```python
from build123d import *

# Parameters (mm, degrees)
SKETCH2_R           = 3.5
BOSS_EXTRUDE1_DEPTH = 3


with BuildPart() as part:
    # Sketch2 → Boss-Extrude1 (new body)
    with BuildSketch(Plane.XY):
        Polygon((-9.966299499, 13.71), (-6.966299499, 13.71), (-6.966299499, 10.71), (-3.966299499, 10.71), (-3.966299499, 13.71), (-0.966299499, 13.71), (-0.966299499, 10.71), (2.033700501, 10.71), (2.033700501, 13.71), (5.033700501, 13.71), (5.033700501, 10.71), (8.033700501, 10.71), (8.033700501, 13.71), (11.033700501, 13.71), (11.033700501, -22.29), (8.033700501, -22.29), (8.033700501, -19.29), (7.033700501, -19.29), (7.033700501, -6.29), (-5.966299499, -6.29), (-5.966299499, -19.29), (-6.966299499, -19.29), (-6.966299499, -22.29), (-9.966299499, -22.29), align=None)
        with Locations((0.533700501, 3.71)):
            Circle(SKETCH2_R, mode=Mode.SUBTRACT)
    extrude(amount=BOSS_EXTRUDE1_DEPTH)


solid = part.part
```
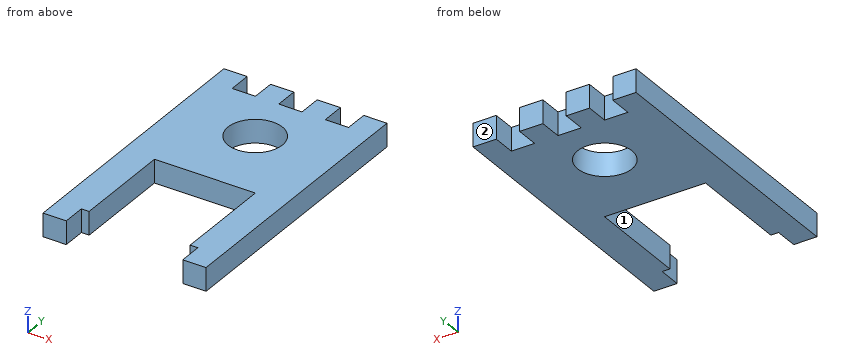
Geometry check sheet. Reference: the model listing, model coordinates, mm. Face numbers are marked on the shaded views. A direction names the side the tool comes from. Coordinates: 2 decimals unless noted, no trailing zeros. Order: outer loops, then holes, each group sorted by start corner. A loop starts at its lowest first (then second) coordinate and runs counter-clockwise, first axis right, second up. Notation, with made-up numbers: (51, 45.25) - (78, 45.25) arc R14 cw to (78, 72.25) - close; hole circle Ø8 at (28, -29). An arc over 180 degrees is marked (long way). Answer in a Markdown table with one row per item. Add a question column.
1. Material ranges on L1, parallel to X at y = 12, z = 0.5; L2, parallel to X at y = -9, z = 2.7; L3, parallel to X at y = 3.5, z = 1.4, recorded low to high. Write a range as [from, to].
2. Section check B-B (z = 1.95). Enter the section's corners in (x, y), plus the area to 3 significant figures.
3. Section check C-C (y = -10.5). Enter the section's corners in (x, z).
4. Access from +Z, -Z, +X, -X, +Y, -Y to the whole of each face (thin tool, end or side, straight path). Record for the marked faces 1 and 2.
5. Gauge pin test, flat ends, axial feed: pin 1 Ø8 at (x, y) = (0.53, 3.71) entering from +Z; pin 2 Ø1 at (x, z) = (-4.5, 0.5) entering from -Y; pin 3 Ø8 at (x, y) = (-0.5, -17) entering from +Z. Record the tip position at first contact, or that the pin passes through.
6. Section check D-D (x = 6.5). Enter the section's corners in (y, z).
7. Section check A-A (y = 3.71). Enter the section's corners in (x, z), plus the area to 3 significant figures.
Data:
| question | item | result |
|---|---|---|
| 1 | L1 | x = [-9.97, -6.97], [-3.97, -0.97], [2.03, 5.03], [8.03, 11.03] |
| 1 | L2 | x = [-9.97, -5.97], [7.03, 11.03] |
| 1 | L3 | x = [-9.97, -2.96], [4.03, 11.03] |
| 2 | outline | (-9.97, -22.29) - (-6.97, -22.29) - (-6.97, -19.29) - (-5.97, -19.29) - (-5.97, -6.29) - (7.03, -6.29) - (7.03, -19.29) - (8.03, -19.29) - (8.03, -22.29) - (11.03, -22.29) - (11.03, 13.71) - (8.03, 13.71) - (8.03, 10.71) - (5.03, 10.71) - (5.03, 13.71) - (2.03, 13.71) - (2.03, 10.71) - (-0.97, 10.71) - (-0.97, 13.71) - (-3.97, 13.71) - (-3.97, 10.71) - (-6.97, 10.71) - (-6.97, 13.71) - (-9.97, 13.71) - close; hole circle Ø7 at (0.53, 3.71) |
| 2 | area | 477 mm² |
| 3 | outline | (-9.97, 0) - (-5.97, 0) - (-5.97, 3) - (-9.97, 3) - close; (7.03, 0) - (11.03, 0) - (11.03, 3) - (7.03, 3) - close |
| 4 | face 1 | +Z, -Z, -Y |
| 4 | face 2 | +Z, -Z, +X, -X, +Y |
| 5 | pin 1 | stops at z = 3 |
| 5 | pin 2 | stops at y = -6.29 |
| 5 | pin 3 | passes through |
| 6 | outline | (-6.29, 0) - (10.71, 0) - (10.71, 3) - (-6.29, 3) - close |
| 7 | outline | (-9.97, 0) - (-2.97, 0) - (-2.97, 3) - (-9.97, 3) - close; (4.03, 0) - (11.03, 0) - (11.03, 3) - (4.03, 3) - close |
| 7 | area | 42.0 mm² |
